from build123d import *

# Parameters (mm, degrees)
SKETCH_2_R          = 3
CUT_EXTRUDE_1_DEPTH = 10
SKETCH_3_R          = 2
CUT_EXTRUDE_2_DEPTH = 24


with BuildPart() as part:
    # Эскиз1 → Повернуть1 (revolve)
    with BuildSketch(Plane.XY):
        Polygon((3.75, 23), (3.75, 3.5), (4.75, 3.5), (4.75, 0), (0, 0), (0, 23), align=None)
    revolve(axis=Axis((0, 0, 0), (0, 1, 0)))

    # Эскиз2 → Вырез-Вытянуть1 (cut)
    with BuildSketch(Plane(origin=(0, 23, 0), x_dir=(1, 0, 0), z_dir=(0, 1, 0))):
        Circle(SKETCH_2_R)
    extrude(amount=-CUT_EXTRUDE_1_DEPTH, mode=Mode.SUBTRACT)

    # Эскиз3 → Вырез-Вытянуть2 (cut, through all)
    with BuildSketch(Plane.XZ):
        Circle(SKETCH_3_R)
    extrude(amount=-CUT_EXTRUDE_2_DEPTH, mode=Mode.SUBTRACT)


solid = part.part
Input: part model. Units: mm. Frame: model coordinates. A direction names the side the tool comes from. Give positions to 0.01 mm unless a question says otherwise; leave off trailing zeros. Write each loop counter-clockwise with the first axis right and the second up, starting at its lowest first coordinate (ties: lowest second). Pieces come first, ordered by that corner, then holes. Notation, with made-up numbers: M -9.75,61 L 18.25,61 A31 ccw 18.25,88 Z; hole C -17,33 d1. An arc over 180 degrees is marked long. Use one line per item in the form item = value.
1. Cut plane C-C on y = 21.75. Return loops of the section in (x, z).
Outcome:
outline = C 0,0 d7.5; hole C 0,0 d6
2. Reachability of faces 1 (the face through (1, 0, 2)), 2 (the face through (1, 13, 2)) from +Z, -Z, +X, -X, +Y, -Y: full face, straight path, thin tool, end or side. Return the list, or none.
Outcome:
face_1 = +Z, -Z, +X, -X, -Y
face_2 = +Y
3. Ray query, L1, parallel to Z at x = 0, y = 17.75; L2, parallel to Z at x = 0, y = 9. Return the intervals inside material, ascending.
Outcome:
L1 = -3.75 to -3, 3 to 3.75
L2 = -3.75 to -2, 2 to 3.75
4. Cut plane A-A on z = 0. Return loops of the section in (x, y), and give its area (3 significant figures).
Outcome:
outline = M -4.75,0 L -2,0 L -2,13 L -3,13 L -3,23 L -3.75,23 L -3.75,3.5 L -4.75,3.5 Z; M 2,0 L 4.75,0 L 4.75,3.5 L 3.75,3.5 L 3.75,23 L 3,23 L 3,13 L 2,13 Z
area = 67.5 mm²
5. Cut plane D-D on x = -3.5. Return loops of the section in (y, z), and give its area (3 significant figures).
Outcome:
outline = M 0,-3.21 L 3.5,-3.21 L 3.5,-1.35 L 23,-1.35 L 23,1.35 L 3.5,1.35 L 3.5,3.21 L 0,3.21 Z
area = 75.0 mm²
6. Mould query, pull axis X, two halves, no side actions, for faces 3 (the face through (0, 6, -2)), 4 (the face through (4, 3.5, 1)), 5 (the face through (-3.746, 13.114, -0.165)). Classes: released by +X, released by -X, zero draft, split by the parting line, or undercut.
Outcome:
face_3 = undercut
face_4 = zero draft
face_5 = split by the parting line
7. Cut plane B-B on x = -0.25. Return loops of the section in (y, z).
Outcome:
outline = M 0,-4.74 L 3.5,-4.74 L 3.5,-3.74 L 23,-3.74 L 23,-2.99 L 13,-2.99 L 13,-1.98 L 0,-1.98 Z; M 0,1.98 L 13,1.98 L 13,2.99 L 23,2.99 L 23,3.74 L 3.5,3.74 L 3.5,4.74 L 0,4.74 Z
8. First-contact query: P1, Ø3.5, axis at x = 0, z = 0, coming from the +Y side; P2, Ø1.5, axis at y = 8, z = 1.5, coming from the +X side; P3, Ø1.5, axis at x = 0.5, y = 16, coming from the -Z side. Flat tips, straight axial feed; report the tip coordinate or a pass-through.
Outcome:
P1 = through
P2 = 3.67
P3 = -3.75
